Geometry: see drawing. Coordinates: mm, zero at the bounding-box minimum. A direction names the side the tool comes from. Give positions to 0.01 mm unless a question says otherwise; leave off trailing zeros. Loops run counter-clockwise (first coordinate to the right, second up) from the corner with the lowest first, then second, coordinate; pieces in that order, holes last. Notation, with made-up numbers: (8.25, 81) -> (51.25, 81) arc R11 ccw to (51.25, 90) -> close; hole circle Ø4 at (-35.75, -7.75). An arc over 180 degrees is marked (long way). Return JSON: item names as keys, results as strings. Group by question number.
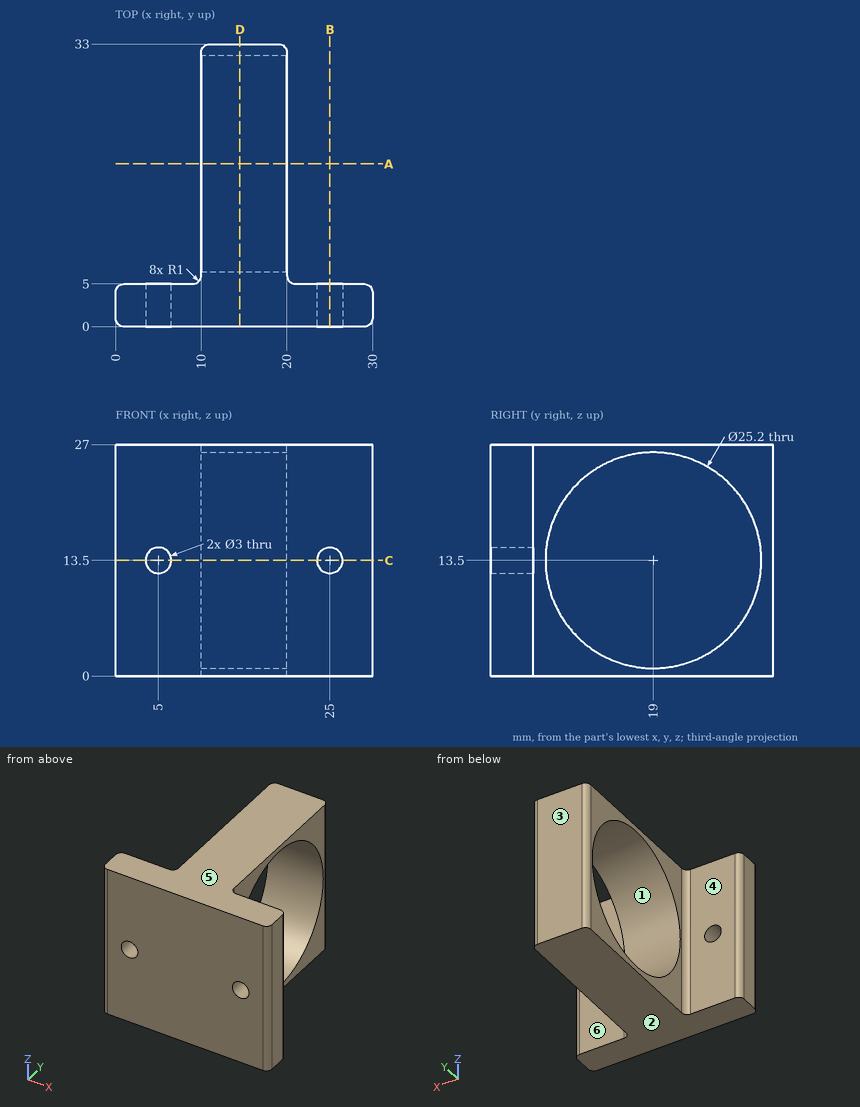
1) Cut plane C-C on z = 13.5. Return loops of the section in (x, y).
2) Mould query, pull axis Y, two halves, no side actions, for the marked faces 1, 2 and 3. Classes: released by +Y, released by -Y, zero draft, split by the parting line, or undercut.
3) Cut plane A-A on y = 19. Return loops of the section in (x, z).
4) Reachability of the marked faces 4, 5 and 6 from +Z, -Z, +X, -X, +Y, -Y: full face, straight path, thin tool, end or side. Return the list, or none.
5) Cut plane D-D on x = 14.5. Return loops of the section in (y, z), then the cut area to 3 significant figures.
6) Cut plane B-B on x = 25. Return loops of the section in (y, z), then the cut area to 3 significant figures.
7) Contact query for a flat-ended pin moving along its axis: P1, Ø2.5, axis at x = 24, z = 18.5, coming from the +Y side. Output: stop coordinate, or through.
8) Material intervals for line 1 (Z direction, x = 17.75, y = 19); line 2 (X direction, y = 9, z = 2); line 3 (Y direction, x = 5, z = 15.5), sorted ascending.
Calculated:
{
 "1": {"outline": "(0, 1) arc R1 ccw to (1, 0) -> (3.5, 0) -> (3.5, 5) -> (1, 5) arc R1 ccw to (0, 4) -> close; (6.5, 0) -> (23.5, 0) -> (23.5, 5) -> (21, 5) arc R1 cw to (20, 6) -> (20, 6.4) -> (10, 6.4) -> (10, 6) arc R1 cw to (9, 5) -> (6.5, 5) -> close; (10, 31.6) -> (20, 31.6) -> (20, 32) arc R1 ccw to (19, 33) -> (11, 33) arc R1 ccw to (10, 32) -> close; (26.5, 0) -> (29, 0) arc R1 ccw to (30, 1) -> (30, 4) arc R1 ccw to (29, 5) -> (26.5, 5) -> close"},
 "2": {"face 1": "undercut", "face 2": "zero draft", "face 3": "released by +Y"},
 "3": {"outline": "(10, 0) -> (20, 0) -> (20, 0.9) -> (10, 0.9) -> close; (10, 26.1) -> (20, 26.1) -> (20, 27) -> (10, 27) -> close"},
 "4": {"face 4": "+Z, -Z, -X, +Y", "face 5": "+Z, +X, -X, +Y, -Y", "face 6": "+Z, -Z, +X, +Y"},
 "5": {"outline": "(0, 0) -> (33, 0) -> (33, 27) -> (0, 27) -> close; hole circle Ø25.2 at (19, 13.5)", "area": "392 mm2"},
 "6": {"outline": "(0, 0) -> (5, 0) -> (5, 12) -> (0, 12) -> close; (0, 15) -> (5, 15) -> (5, 27) -> (0, 27) -> close", "area": "120 mm2"},
 "7": {"P1": "y = 5"},
 "8": {"line 1": "0 to 0.9, 26.1 to 27", "line 2": "10 to 20", "line 3": "0 to 5"}
}
